Here's how the part is built. I have some questions about the finished solid (model axes, mm). Round coordinates to 2 decimals unless told otherwise and drop trailing zeros. Write each loop counter-clockwise with the first axis right and the second up, starting at its lowest first coordinate (ties: lowest second). Pieces come first, ordered by that corner, then holes. Notation, with made-up numbers: (55.5, 57.5) -> (109.5, 57.5) arc R7 cw to (109.5, 62.5) -> close; hole circle Ø6 at (48, -1). An arc over 180 degrees is marked (long way). Answer in a Markdown table with one row per item. Add a question column.
from build123d import *

# Parameters (mm, degrees)
ESBO_O1_W                = 24
ESBO_O1_H                = 17
ESBO_O1_R                = 1.5
RESSALTO_EXTRUS_O1_DEPTH = 1
FILETE1_R                = 3


with BuildPart() as part:
    # Esboço1 → Ressalto-extrusão1 (new, symmetric)
    with BuildSketch(Plane.XY):
        Rectangle(ESBO_O1_W, ESBO_O1_H)
        with Locations((-9, 5.5)):
            Circle(ESBO_O1_R, mode=Mode.SUBTRACT)
        with Locations(Location((9, 5.5, 0), (0, 0, 180))):
            Circle(ESBO_O1_R, mode=Mode.SUBTRACT)
        with Locations((9, -5.5)):
            Circle(ESBO_O1_R, mode=Mode.SUBTRACT)
        with Locations(Location((-9, -5.5, 0), (0, 0, 180))):
            Circle(ESBO_O1_R, mode=Mode.SUBTRACT)
    extrude(amount=RESSALTO_EXTRUS_O1_DEPTH, both=True)

    # Filete1
    filete1_edges = [part.edges().sort_by_distance(p)[0] for p in [
        (12, -8.5, 0),
        (-12, -8.5, 0),
        (-12, 8.5, 0),
        (12, 8.5, 0),
    ]]
    fillet(filete1_edges, radius=FILETE1_R)


solid = part.part
Item 1: I need wall thicknesses on line 1 along Y through (x, z) = (9, 0.15); line 2 along X through (y, z) = (-5.25, 0.3); line 3 along X through (y, z) = (5, 0.9). Which ranges of each line are inside material? Lowest first, please. Write a range as from..to.
Item 2: For P1, Ø2.5, axis at x = 9, y = 5.5, coming from the +Z side, with a flat end and sliding along its axis, tell me the tip position at first contact or that it passes through.
Item 3: If we section it at B-B on z = -0.25: Please give me the cut outline in (x, y).
Item 4: If we section it at C-C on x = -9.25: Please give me the cut outline in (y, z), then the cut area to 3 significant figures.
Item 5: If we section it at A-A on y = -6.25: Please give me the cut outline in (x, z).
Item 6: If we mould it in two halves opening along Y, with no side actions, what happens to faces 1 (the cylindrical face through (11.14, 7.6, -0.01)), 2 (the flat face through (0, 0, -1)), 3 (the cylindrical face through (-10.5, 5.57, -0.01)), 4 (the cylindrical face through (10.5, 5.43, -0.01))? For each: pulls with the +Y half, pulls with the -Y half, needs draft (parallel to the pull), parting line crosses it, or undercut.
Results list:
| question | item | result |
|---|---|---|
| 1 | line 1 | -8.5..-7, -4..4, 7..8.5 |
| 1 | line 2 | -12..-10.48, -7.52..7.52, 10.48..12 |
| 1 | line 3 | -12..-10.41, -7.59..7.59, 10.41..12 |
| 2 | P1 | through |
| 3 | outline | (-12, -5.5) arc R3 ccw to (-9, -8.5) -> (9, -8.5) arc R3 ccw to (12, -5.5) -> (12, 5.5) arc R3 ccw to (9, 8.5) -> (-9, 8.5) arc R3 ccw to (-12, 5.5) -> close; hole circle Ø3 at (-9, -5.5); hole circle Ø3 at (-9, 5.5); hole circle Ø3 at (9, -5.5); hole circle Ø3 at (9, 5.5) |
| 4 | outline | (-8.49, -1) -> (-6.98, -1) -> (-6.98, 1) -> (-8.49, 1) -> close; (-4.02, -1) -> (4.02, -1) -> (4.02, 1) -> (-4.02, 1) -> close; (6.98, -1) -> (8.49, -1) -> (8.49, 1) -> (6.98, 1) -> close |
| 4 | area | 22.1 mm² |
| 5 | outline | (-11.9, -1) -> (-10.3, -1) -> (-10.3, 1) -> (-11.9, 1) -> close; (-7.7, -1) -> (7.7, -1) -> (7.7, 1) -> (-7.7, 1) -> close; (10.3, -1) -> (11.9, -1) -> (11.9, 1) -> (10.3, 1) -> close |
| 6 | face 1 | pulls with the +Y half |
| 6 | face 2 | needs draft |
| 6 | face 3 | undercut |
| 6 | face 4 | undercut |
